Autodesk Inventor part; units mm, degrees
ref_plane "YZ Plane" through (0, 0, 0) normal (1, 0, 0) x (0, 1, 0)
ref_plane "XZ Plane" through (0, 0, 0) normal (0, 1, 0) x (-1, 0, 0)
ref_plane "XY Plane" through (0, 0, 0) normal (0, 0, 1) x (1, 0, 0)
sketch "スケッチ1" plane through (0, 0, 0) normal (0, 0, 1) x (1, 0, 0)
  line L0 (-2.0207, 3.5) -> (2.0207, 3.5)
  line L1 (2.0207, 3.5) -> (4.0415, 0)
  line L2 (4.0415, 0) -> (2.0207, -3.5)
  line L3 (2.0207, -3.5) -> (-2.0207, -3.5)
  line L4 (-2.0207, -3.5) -> (-4.0415, 0)
  line L5 (-4.0415, 0) -> (-2.0207, 3.5)
  circle A0 centre (0, 0) radius 2
  dimension "d0" = 7
  dimension "d1" = 4
extrude "押し出し1" add sketch "スケッチ1" along normal blind 5.5
sketch "スケッチ2" plane through (0, 0, 5.5) normal (0, 0, 1) x (1, 0, 0)
  line L0 (2.0207, 3.5) -> (-2.0207, 3.5)
  line L1 (-2.0207, 3.5) -> (-4.0415, 0)
  line L2 (-4.0415, 0) -> (-2.0207, -3.5)
  line L3 (-2.0207, -3.5) -> (2.0207, -3.5)
  line L4 (2.0207, -3.5) -> (4.0415, 0)
  line L5 (4.0415, 0) -> (2.0207, 3.5)
  circle A0 centre (0, 0) radius 3.5
extrude "押し出し2" cut sketch "スケッチ2" against normal blind 1 contours L5 A0 L0 | A0 L1 L0 | L5 L4 A0 | A0 L2 L1 | A0 L3 L2 | L4 L3 A0
properties part number "ナイロンナットm4" material "鋼、高強度、低合金"
Can you work these out from the model? Positions are in its coordinate system, mm. A direction names the side the tool comes from. Coordinates: 2 decimals unless noted, no trailing zeros. Write each loop counter-clockwise with the first axis right and the second up, starting at its lowest first coordinate (ties: lowest second). Pieces come first, ordered by that corner, then holes. Notation, with made-up numbers: (47.5, 29.5) -> (100.5, 29.5) arc R27 cw to (100.5, 46.5) -> close; hole circle Ø6 at (-31.5, 40.25). An arc over 180 degrees is marked (long way). Write each question's results on one line, items separated by ' | '. Start each with the question number.
Item 1: I'm going to push a flat-ended pin straight in: P1, Ø1, axis at x = 3, z = 1.5, coming from the -Y side. Where does the tip first touch, or does it pass through?
Item 2: Please list where these lines run through material, in increasing order: probe 1 along Y at (x, z) = (0, 3.25); probe 2 along X at (y, z) = (-0.25, 2.6); probe 3 along X at (y, z) = (1.75, 4.4).
Item 3: If we section it at C-C, the plane x = -1.5: Write out the boundary of the cut face in (y, z), and give its area (3 significant figures).
Item 4: Thinking about a two-plate mould opening in X: for faces 4 (the flat face through (-3.045, 1.726, 2.218)), 5 (the cylindrical face through (1.05, -3.34, 5.01)), 6 (the flat face through (0, 3.5, 2)), 7 (the cylindrical face through (0, 2, 3)), which applies, released by +X, released by -X, zero draft, split by the parting line, or undercut?
Item 5: On a 3-axis mill with a long thin cutter (end or side, diameter ignored), from which of +Z, -Z, +X, -X, +Y, -Y can I reach the whole of each face in a straight line? I mean faces 1 (the flat face through (-1.86, 3.15, 4.5)), 2 (the flat face through (1.85, 3.15, 4.5)), 3 (the flat face through (-1.9, -3.2, 4.5)). Say none if no direction works.
Item 6: If we section it at B-B, the plane y = -0.25: Write out the boundary of the cut face in (x, z), and give its area (3 significant figures).
Item 7: If we section it at A-A, the plane z = 1.4: Write out the boundary of the cut face in (x, y).
Item 8: If we section it at D-D, the plane y = -2.75: Write out the boundary of the cut face in (x, z).
Answer block:
1) P1: y = -2.67
2) probe 1: -3.5 to -2, 2 to 3.5 | probe 2: -3.9 to -1.98, 1.98 to 3.9 | probe 3: -3.03 to -0.97, 0.97 to 3.03
3) outline: (-3.5, 0) -> (-1.32, 0) -> (-1.32, 5.5) -> (-3.16, 5.5) -> (-3.16, 4.5) -> (-3.5, 4.5) -> close; (1.32, 0) -> (3.5, 0) -> (3.5, 4.5) -> (3.16, 4.5) -> (3.16, 5.5) -> (1.32, 5.5) -> close | area: 23.3 mm²
4) face 4: released by -X | face 5: split by the parting line | face 6: zero draft | face 7: undercut
5) face 1: +Z, -X, +Y | face 2: +Z, +X, +Y | face 3: +Z, -X, -Y
6) outline: (-3.9, 0) -> (-1.98, 0) -> (-1.98, 5.5) -> (-3.49, 5.5) -> (-3.49, 4.5) -> (-3.9, 4.5) -> close; (1.98, 0) -> (3.9, 0) -> (3.9, 4.5) -> (3.49, 4.5) -> (3.49, 5.5) -> (1.98, 5.5) -> close | area: 20.2 mm²
7) outline: (-4.04, 0) -> (-2.02, -3.5) -> (2.02, -3.5) -> (4.04, 0) -> (2.02, 3.5) -> (-2.02, 3.5) -> close; hole circle Ø4 at (0, 0)
8) outline: (-2.45, 0) -> (2.45, 0) -> (2.45, 4.5) -> (2.17, 4.5) -> (2.17, 5.5) -> (-2.17, 5.5) -> (-2.17, 4.5) -> (-2.45, 4.5) -> close
